```python
from build123d import *
from build123d.topology import SkipClean

# Parameters (mm, degrees)
PROFILEBOSS_EXTRUDE1_DEPTH           = 33
SKETCH2_OUTSIDE_W                    = 43.906
SKETCH2_OUTSIDE_H                    = 23.206
SIDEPROFILECUT_EXTRUDE1_DEPTH        = 45.529231972
SKETCH3_W                            = 11.132045058
SKETCH3_H                            = 23.65
BOTTOMCUT_EXTRUDE2_DEPTH             = 44.795576261
DRAGLINKMOUNTHOLESSKETCH4_R          = 2
DRAGLINKMOUNTHOLESCUT_EXTRUDE3_DEPTH = 44.795576261
CHAMFER1_SIZE                        = 1.5
CHAMFER1_SIZE2                       = 0.97411139
RIGHTINNERBOSS_EXTRUDE3_START        = 1.85
RIGHTINNERBOSS_EXTRUDE3_DEPTH        = 1.85
LEFTINNERBOSS_EXTRUDE4_DEPTH         = 1.85
RIGHTOUTERCIRCLESKETCH7_R            = 2.5
RIGHTOUTERCIRCLECUT_EXTRUDE4_DEPTH   = 1.85
LEFTOUTERCIRCLECUT_EXTRUDE5_START    = -1.85
SKETCH8_R                            = 2.475
LEFTOUTERCIRCLECUT_EXTRUDE5_DEPTH    = 1.85
CHAMFER2_SIZE                        = 1.85


with BuildPart() as part:
    # Sketch1 → ProfileBoss-Extrude1 (new body)
    with BuildSketch(Plane(origin=(0, 0, 0), x_dir=(0, 0, -1), z_dir=(1, 0, 0))):
        Polygon((0, 12.3), (0, 0), (27.25, 0), (27.25, 12.3), (25.45, 12.3), (25.45, 3), (1.8, 3), (1.8, 12.3), align=None)
    extrude(amount=PROFILEBOSS_EXTRUDE1_DEPTH)

    # Sketch2 outside → SideProfileCut-Extrude1 (cut, through all)
    with BuildSketch(Plane.XY):
        with Locations((16.5, 6.15)):
            Rectangle(SKETCH2_OUTSIDE_W, SKETCH2_OUTSIDE_H)
        with BuildLine():
            Line((14.789600469, 12.3), (33, 6))
            Line((33, 6), (33, 0))
            Line((33, 0), (6.15, 0))
            ThreePointArc((6.15, 0), (0.000396167, 6.219804731), (6.289600469, 12.298415382))
            Line((6.289600469, 12.298415382), (14.789600469, 12.3))
        make_face(mode=Mode.SUBTRACT)
    extrude(amount=-SIDEPROFILECUT_EXTRUDE1_DEPTH, mode=Mode.SUBTRACT)

    # Sketch3 → BottomCut-Extrude2 (cut, through all)
    with BuildSketch(Plane(origin=(0, 3, 0), x_dir=(1, 0, 0), z_dir=(0, 1, 0))):
        with Locations((6.433977471, 13.625)):
            Rectangle(SKETCH3_W, SKETCH3_H)
    extrude(amount=-BOTTOMCUT_EXTRUDE2_DEPTH, mode=Mode.SUBTRACT)

    # DragLinkMountHolesSketch4 → DragLinkMountHolesCut-Extrude3 (cut, through all)
    with BuildSketch(Plane(origin=(0, 3, 0), x_dir=(1, 0, 0), z_dir=(0, 1, 0))):
        with Locations(Location((28, 19.625, 0), (0, 0, 270))):
            Circle(DRAGLINKMOUNTHOLESSKETCH4_R)
        with Locations(Location((28, 7.625, 0), (0, 0, 270))):
            Circle(DRAGLINKMOUNTHOLESSKETCH4_R)
        with Locations(Location((20.5, 13.625, 0), (0, 0, 270))):
            Circle(DRAGLINKMOUNTHOLESSKETCH4_R)
    extrude(amount=-DRAGLINKMOUNTHOLESCUT_EXTRUDE3_DEPTH, mode=Mode.SUBTRACT)

    # Chamfer1
    chamfer1_edges = [part.edges().sort_by_distance(p)[0] for p in [
        (28, 3, -21.625),
        (28, 3, -9.625),
        (20.5, 3, -15.625),
    ]]
    chamfer1_side = [part.faces().sort_by_distance(p)[0] for p in [
        (12.316278754, 3, -13.625),
    ]]
    chamfer(chamfer1_edges, length=CHAMFER1_SIZE, length2=CHAMFER1_SIZE2, reference=chamfer1_side[0])

    # Sketch11 → RightInnerBoss-Extrude3 (add)
    with BuildSketch(Plane.XY.offset(-25.45).offset(RIGHTINNERBOSS_EXTRUDE3_START)):
        with BuildLine():
            Line((14.789600469, 12.3), (6.15, 12.3))
            ThreePointArc((6.15, 12.3), (0, 6.15), (6.15, 0))
            Line((6.15, 0), (14.789600469, 0))
            Line((14.789600469, 0), (14.789600469, 12.3))
        make_face()
    extrude(amount=-RIGHTINNERBOSS_EXTRUDE3_DEPTH)

    # Sketch12 → LeftInnerBoss-Extrude4 (add)
    with SkipClean():  # the faces are left unmerged after this step: merging them gives an invalid solid
        with BuildSketch(Plane(origin=(0, 0, -1.8), x_dir=(-1, 0, 0), z_dir=(0, 0, -1))):
            with BuildLine():
                Line((-14.789600469, 12.3), (-6.289600469, 12.298415382))
                ThreePointArc((-6.289600469, 12.298415382), (-0.000396167, 6.219804731), (-6.15, 0))
                Line((-6.15, 0), (-14.789600469, 0))
                Line((-14.789600469, 0), (-14.789600469, 12.3))
            make_face()
        extrude(amount=LEFTINNERBOSS_EXTRUDE4_DEPTH)

    # RightOuterCircleSketch7 → RightOuterCircleCut-Extrude4 (cut)
    with SkipClean():  # the faces are left unmerged after this step: merging them gives an invalid solid
        with BuildSketch(Plane(origin=(0, 0, -27.25), x_dir=(-1, 0, 0), z_dir=(0, 0, -1))):
            with BuildLine():
                Line((-13.55, 12.299768907), (-10.266779115, 12.29915683))
                ThreePointArc((-10.266779115, 12.29915683), (1.249999961, 6.150757924), (-10.265519408, 0))
                Line((-10.265519408, 0), (-13.55, 0))
                Line((-13.55, 0), (-13.55, 12.299768907))
            make_face()
            with Locations((-6.15, 6.15)):
                Circle(RIGHTOUTERCIRCLESKETCH7_R, mode=Mode.SUBTRACT)
        extrude(amount=-RIGHTOUTERCIRCLECUT_EXTRUDE4_DEPTH, mode=Mode.SUBTRACT)

    # Sketch8 → LeftOuterCircleCut-Extrude5 (cut)
    with BuildSketch(Plane.XY.offset(LEFTOUTERCIRCLECUT_EXTRUDE5_START)):
        with BuildLine():
            Line((13.550000004, 12.299768907), (10.266779119, 12.29915683))
            ThreePointArc((10.266779119, 12.29915683), (-1.249999964, 6.150757924), (10.265519413, 0))
            Line((10.265519413, 0), (13.548740355, 0))
            Line((13.548740355, 0), (13.550000004, 12.299768907))
        make_face()
        with Locations((6.15, 6.15)):
            Circle(SKETCH8_R, mode=Mode.SUBTRACT)
    extrude(amount=LEFTOUTERCIRCLECUT_EXTRUDE5_DEPTH, mode=Mode.SUBTRACT)

    # Chamfer2
    chamfer2_edges = [part.edges().sort_by_distance(p)[0] for p in [
        (14.789600469, 7.65, -23.6),
        (14.789600469, 7.65, -3.65),
    ]]
    chamfer(chamfer2_edges, length=CHAMFER2_SIZE - 0.0001)  # a hair under: the kernel refuses the full size


solid = part.part
```
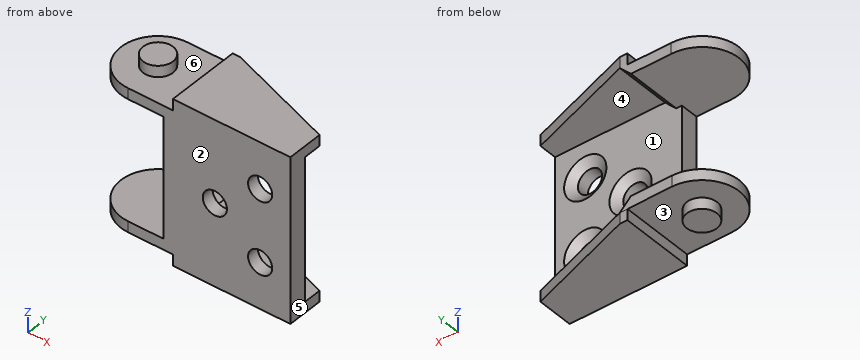
Geometry check sheet. Reference: the model listing, model coordinates, mm. Face numbers are marked on the shaded views. A direction names the side the tool comes from. Round coordinates to 2 decimals unless told otherwise and drop trailing zeros. Loops run counter-clockwise (first coordinate to the right, second up) from the corner with the lowest first, then second, coordinate; pieces in that order, holes last. Notation, with made-up numbers: M 4.25,11 L 13.25,11 A31 cw 13.25,37 Z; hole C -12,-18 d7. An arc over 180 degrees is marked long. Return JSON: item names as keys, results as strings. Group by question number.
(1) Scan lines: line 1 along Z through (x, y) = (4, 6); line 2 along Z through (x, y) = (29, 6); line 3 along Y through (x, z) = (16.5, -4.5). Record each from-to range of solid material in increasing order. Write a range as [from, to].
(2) Section check D-D, the plane y = 1.25. Enter the section's corners in (x, z) (3 decimals).
(3) Set-up check for the marked faces 1, 2 and 3: record each of +Z, -Z, +X, -X, +Y, -Y from which the full face is reachable in a straight line by a thin tool's end or side.
(4) Section check B-B, the plane x = 20.5. Enter the section's corners in (y, z) (3 decimals).
(5) Mould release check, pull along X, two halves, no side actions. Record for the marked faces 4, 5 and 6: pulls with the +X half, pulls with the -X half, needs draft (parallel to the pull), parting line crosses it, or undercut.
(6) Section check C-C, the plane x = 28. Enter the section's corners in (y, z) (3 decimals).
(7) Go/stop test with flat-tipped pins: pin 1 (4 mm diameter, centred on x = 4.5, z = -22, fed in from +Y); pin 2 (5 mm diameter, centred on y = 9.5, z = -4.5, fed in from +X); pin 3 (3 mm diameter, centred on x = 19, z = -4.5, fed in from +Y). Record where each tip stops, or that it passes through.
Data:
{
 "1": {"line 1": "[-27.25, -23.6], [-3.65, 0]", "line 2": "[-27.25, -25.45], [-1.8, 0]", "line 3": "[0, 3]"},
 "2": {"outline": "M 2.433,-25.4 L 13.55,-25.4 L 13.55,-27.25 L 33,-27.25 L 33,0 L 13.549,0 L 13.549,-1.85 L 2.433,-1.85 L 2.433,-3.65 L 12,-3.65 L 12,-23.6 L 2.433,-23.6 Z; hole C 20.5,-13.625 d4; hole C 28,-19.625 d4; hole C 28,-7.625 d4"},
 "3": {"face 1": "+X, +Y", "face 2": "+Z, -Z, +X, -X, -Y", "face 3": "-Z"},
 "4": {"outline": "M 0,-27.25 L 10.324,-27.25 L 10.324,-25.45 L 3,-25.45 L 3,-17.125 L 2.026,-15.625 L 0,-15.625 Z; M 0,-11.625 L 2.026,-11.625 L 3,-10.125 L 3,-1.8 L 10.324,-1.8 L 10.324,0 L 0,0 Z"},
 "5": {"face 4": "needs draft", "face 5": "pulls with the +X half", "face 6": "undercut"},
 "6": {"outline": "M 0,-27.25 L 7.73,-27.25 L 7.73,-25.45 L 3,-25.45 L 3,-23.125 L 2.026,-21.625 L 0,-21.625 Z; M 0,-17.625 L 2.026,-17.625 L 3,-16.125 L 3,-11.125 L 2.026,-9.625 L 0,-9.625 Z; M 0,-5.625 L 2.026,-5.625 L 3,-4.125 L 3,-1.8 L 7.73,-1.8 L 7.73,0 L 0,0 Z"},
 "7": {"pin 1": "y = 12.28", "pin 2": "x = 14.59", "pin 3": "y = 3"}
}
